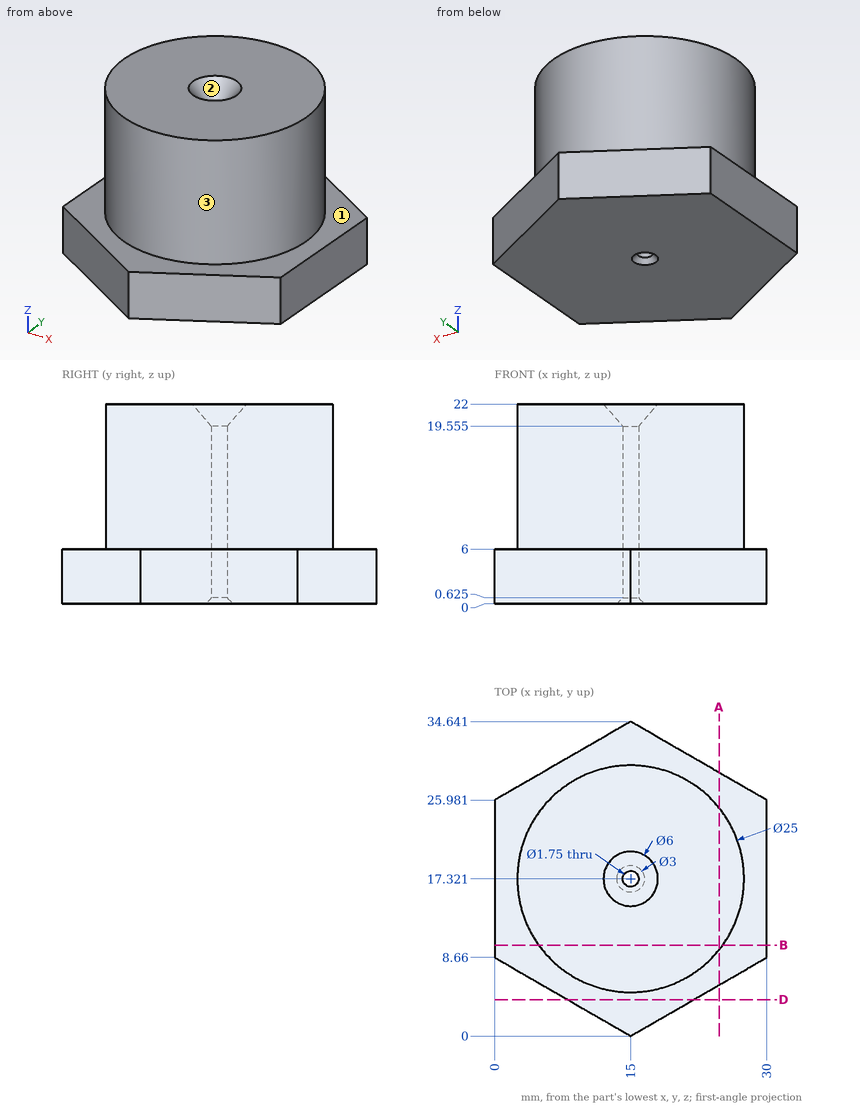
Check sheet for the drawn part. Datum: minimum x, y, z corner. Units: mm. Round coordinates to 2 decimals unless told otherwise and drop trailing zeros. Order: outer loops, then holes, each group sorted by start corner. A loop starts at its lowest first (then second) coordinate and runs counter-clockwise, first axis right, second up. Notation, with made-up numbers: M -23.5,75 L -9.5,75 A28 cw -9.5,114 Z; hole C 81,16 d2. An arc over 180 degrees is marked long. Write each question's results on one line, items separated by ' | '. Start each with the question number.
1. Cross-section at B-B on y = 10. Record the boundary of the cut face in (x, z), plus the area to 3 significant figures.
2. Draft check along X on the marked faces 1, 2 and 3. Enter one of: pulls with the +X half, pulls with the -X half, needs draft (parallel to the pull), parting line crosses it, or undercut.
3. Go/stop test with flat-tipped pins: P1, Ø6, axis at x = 10.5, z = 16.5, coming from the -Y side; P2, Ø1.5, axis at x = 26.5, z = 5, coming from the +Y side (1 decimal); P3, Ø2, axis at y = 26.5, z = 11, coming from the +X side. Record where each tip stops, or that it passes through.
4. Cross-section at D-D on y = 4. Record the boundary of the cut face in (x, z).
5. Cross-section at A-A on x = 24.75. Record the boundary of the cut face in (y, z), plus the area to 3 significant figures.
6. Material ranges on L1, parallel to Y at x = 15, z = 4.5 (1 decimal); L2, parallel to Y at x = 15, z = 15 (1 decimal); L3, parallel to Z at x = 19.75, y = 5, recorded low to high. Write a range as from..to.
Resolved:
1) outline: M 0,0 L 30,0 L 30,6 L 25.13,6 L 25.13,22 L 4.87,22 L 4.87,6 L 0,6 Z | area: 504 mm2
2) face 1: needs draft | face 2: undercut | face 3: parting line crosses it
3) P1: y = 4.91 | P2: y = 28.4 | P3: x = 24.45
4) outline: M 8.07,0 L 21.93,0 L 21.93,6 L 8.07,6 Z
5) outline: M 5.63,0 L 29.01,0 L 29.01,6 L 25.14,6 L 25.14,22 L 9.5,22 L 9.5,6 L 5.63,6 Z | area: 391 mm2
6) L1: 0..16.4, 18.2..34.6 | L2: 4.8..16.4, 18.2..29.8 | L3: 0..6
